Autodesk Inventor part; units mm, degrees
ref_plane "YZ Plane" through (0, 0, 0) normal (1, 0, 0) x (0, 1, 0)
ref_plane "XZ Plane" through (0, 0, 0) normal (0, 1, 0) x (-1, 0, 0)
ref_plane "XY Plane" through (0, 0, 0) normal (0, 0, 1) x (1, 0, 0)
sketch "Sketch1" plane through (0, 0, 0) normal (0, 0, 1) x (1, 0, 0)
  line L0 (-25.4, -12.7) -> (25.4, -12.7)
  line L1 (25.4, -12.7) -> (25.4, 12.7)
  line L2 (25.4, 12.7) -> (-25.4, 12.7)
  line L3 (-25.4, 12.7) -> (-25.4, -12.7)
  line L4 (-25.4, -12.7) -> (25.4, 12.7) construction
  line L5 (25.4, -12.7) -> (-25.4, 12.7) construction
  point P0 (0, 0)
  dimension "d0" = 25.4
  dimension "d1" = 50.8
extrude "Extrusion1" add sketch "Sketch1" against normal blind 304.8
sketch "Sketch2" plane through (-25.4, 12.7, 0) normal (0, 1, 0) x (1, 0, 0)
  circle A0 centre (25.4, 63.5) radius 9.525
  circle A1 centre (25.4, 241.3) radius 9.525
  line L0 (50.8, 0) -> (0, 0)
  line L1 (0, 0) -> (0, 304.8)
  point P0 (25.4, 0)
  point P1 (25.4, 0)
  point P2 (0, 152.4)
  dimension "d4" = 177.8
  dimension "d5" = 88.9
  dimension "d6" = 19.05
extrude "Extrusion2" cut sketch "Sketch2" against normal blind 254
properties part number "Metal Bar-1"
Work out the finished part from the listing and answer in its coordinate system (mm). Coordinates: 2 decimals unless noted, no trailing zeros. Write each loop counter-clockwise with the first axis right and the second up, starting at its lowest first coordinate (ties: lowest second). Pieces come first, ordered by that corner, then holes.
Q1. Determine the mould class of faces 1 (the face through (0, -12.7, -150)), 2 (the face through (0, 0, -304.8)), 3 (the face through (-7.02, 0.18, -69.94)) for opening direction Z: released by +Z, released by -Z, zero draft, split by the parting line, or undercut.
Q2. Find the intervals of material crossed by line 1 (Z direction, x = 0, y = 2.5) (3 decimals); line 2 (X direction, y = 1, z = -241.3) (3 decimals); line 3 (Z direction, x = 5, y = -8.25), in increasing order.
Q3. A cutting plane is placed at C-C, the plane y = 2. Give the vertices of the cut face in (x, z) (3 decimals).
Q4. A cutting plane is placed at B-B, the plane z = -241.3. Give the vertices of the cut face in (x, y) (3 decimals), then the cut area to 3 significant figures.
Q5. This flat-tipped pin is pushed along its axis until it touches: pin 1 Ø15 at (x, z) = (0, -63.5) entering from -Y. Where does it stop, or does it pass through?
Q6. A cutting plane is placed at A-A, the plane x = 0. Give the vertices of the cut face in (y, z) (3 decimals), then the cut area to 3 significant figures.
Findings below:
1. face 1: zero draft
1. face 2: released by -Z
1. face 3: undercut
2. line 1: z = -304.8 to -250.825, -231.775 to -73.025, -53.975 to 0
2. line 2: x = -25.4 to -9.525, 9.525 to 25.4
2. line 3: z = -304.8 to -249.41, -233.19 to -71.61, -55.39 to 0
3. outline: (-25.4, -304.8) - (25.4, -304.8) - (25.4, 0) - (-25.4, 0) - close; hole circle Ø19.05 at (0, -241.3); hole circle Ø19.05 at (0, -63.5)
4. outline: (-25.4, -12.7) - (-9.525, -12.7) - (-9.525, 12.7) - (-25.4, 12.7) - close; (9.525, -12.7) - (25.4, -12.7) - (25.4, 12.7) - (9.525, 12.7) - close
4. area: 806 mm2
5. pin 1: passes through
6. outline: (-12.7, -304.8) - (12.7, -304.8) - (12.7, -250.825) - (-12.7, -250.825) - close; (-12.7, -231.775) - (12.7, -231.775) - (12.7, -73.025) - (-12.7, -73.025) - close; (-12.7, -53.975) - (12.7, -53.975) - (12.7, 0) - (-12.7, 0) - close
6. area: 6,770 mm2
